Build history of the part. All positions in model axes, mm. Face numbers are marked on the shaded views. A direction names the side the tool comes from. Round coordinates to 2 decimals unless told otherwise and drop trailing zeros. Write each loop counter-clockwise with the first axis right and the second up, starting at its lowest first coordinate (ties: lowest second). Pieces come first, ordered by that corner, then holes.
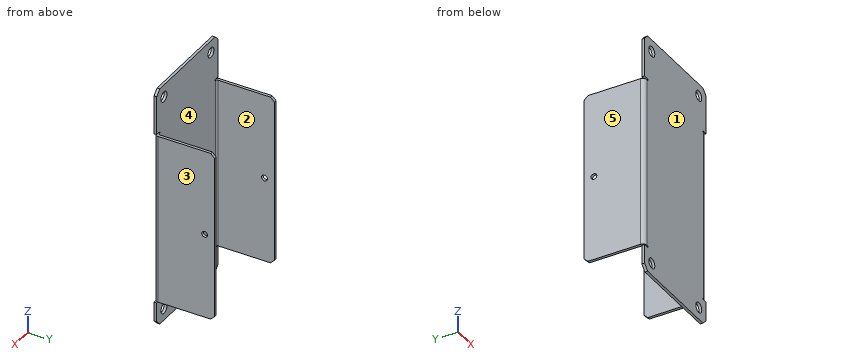
from build123d import *

# Parameters (mm, degrees)
SKETCH1_W                       = 53.65
SKETCH1_H                       = 124.45
SKETCH1_R                       = 2.61
BASE_FLANGE1_DEPTH              = 1.4
CHAMFER1_SIZE                   = 2.7
EDGE_FLANGE2_STRIP_W            = 7.0732
EDGE_FLANGE2_STRIP_H            = 1.4
EDGE_FLANGE2_STRIP_CUT_DEPTH    = 87.7
EDGE_FLANGE2_RELIEF_W           = 7.7732
EDGE_FLANGE2_RELIEF_H           = 0.7
EDGE_FLANGE2_RELIEF_CUT_DEPTH   = 1.4
EDGE_FLANGE2_STRIP_2_W          = 7.0732
EDGE_FLANGE2_STRIP_2_H          = 1.4
EDGE_FLANGE2_STRIP_CUT_2_DEPTH  = 87.7
EDGE_FLANGE2_RELIEF_2_W         = 7.7732
EDGE_FLANGE2_RELIEF_2_H         = 0.7
EDGE_FLANGE2_RELIEF_CUT_2_DEPTH = 1.4
EDGE_FLANGE2_DEPTH              = 87.7
EDGE_FLANGE2_BEND_DEPTH         = 87.7
CHAMFER2_SIZE                   = 2
SKETCH18_R                      = 1.5
CUT_EXTRUDE1_DEPTH              = 88.329451647


# Sheet-metal steps are written as plain solids
with BuildPart() as part:
    # Sketch1 → Base-Flange1 (new body)
    with BuildSketch(Plane(origin=(0, 0, 0), x_dir=(1, 0, 0), z_dir=(0, 1, 0))):
        Rectangle(SKETCH1_W, SKETCH1_H)
        with Locations(Location((-20.5, 56, 0), (0, 0, 270))):
            Circle(SKETCH1_R, mode=Mode.SUBTRACT)
        with Locations(Location((20.5, 56, 0), (0, 0, 270))):
            Circle(SKETCH1_R, mode=Mode.SUBTRACT)
        with Locations(Location((20.5, -56, 0), (0, 0, 270))):
            Circle(SKETCH1_R, mode=Mode.SUBTRACT)
        with Locations(Location((-20.5, -56, 0), (0, 0, 270))):
            Circle(SKETCH1_R, mode=Mode.SUBTRACT)
    extrude(amount=-BASE_FLANGE1_DEPTH)

    # Chamfer1
    chamfer1_edges = [part.edges().sort_by_distance(p)[0] for p in [
        (26.825, -0.7, 62.225),
        (-26.825, -0.7, 62.225),
        (-26.825, -0.7, -62.225),
        (26.825, -0.7, -62.225),
    ]]
    chamfer(chamfer1_edges, length=CHAMFER1_SIZE)

    # Edge-Flange2 strip (across the edge) → Edge-Flange2 strip cut (cut)
    with BuildSketch(Plane(origin=(26.825, 0, 38.825), x_dir=(-1, 0, 0), z_dir=(0, 0, -1))):
        with Locations((-1.4, -0.7)):
            Rectangle(EDGE_FLANGE2_STRIP_W, EDGE_FLANGE2_STRIP_H)
    extrude(amount=EDGE_FLANGE2_STRIP_CUT_DEPTH, mode=Mode.SUBTRACT)

    # Edge-Flange2 relief (on the sheet) → Edge-Flange2 relief cut (cut)
    with BuildSketch(Plane(origin=(24.6884, 0, 38.825), x_dir=(-1, 0, 0), z_dir=(0, 1, 0))):
        with Locations((-3.1866, 0.35)):
            Rectangle(EDGE_FLANGE2_RELIEF_W, EDGE_FLANGE2_RELIEF_H)
        with Locations((-3.1866, -88.05)):
            Rectangle(EDGE_FLANGE2_RELIEF_W, EDGE_FLANGE2_RELIEF_H)
    extrude(amount=-EDGE_FLANGE2_RELIEF_CUT_DEPTH, mode=Mode.SUBTRACT)

    # Edge-Flange2 strip 2 (across the edge) → Edge-Flange2 strip cut 2 (cut)
    with BuildSketch(Plane(origin=(-26.825, 0, -48.875), x_dir=(1, 0, 0), z_dir=(0, 0, 1))):
        with Locations((-1.4, -0.7)):
            Rectangle(EDGE_FLANGE2_STRIP_2_W, EDGE_FLANGE2_STRIP_2_H)
    extrude(amount=EDGE_FLANGE2_STRIP_CUT_2_DEPTH, mode=Mode.SUBTRACT)

    # Edge-Flange2 relief 2 (on the sheet) → Edge-Flange2 relief cut 2 (cut)
    with BuildSketch(Plane(origin=(-24.6884, 0, -48.875), x_dir=(1, 0, 0), z_dir=(0, 1, 0))):
        with Locations((-3.1866, 0.35)):
            Rectangle(EDGE_FLANGE2_RELIEF_2_W, EDGE_FLANGE2_RELIEF_2_H)
        with Locations((-3.1866, -88.05)):
            Rectangle(EDGE_FLANGE2_RELIEF_2_W, EDGE_FLANGE2_RELIEF_2_H)
    extrude(amount=-EDGE_FLANGE2_RELIEF_CUT_2_DEPTH, mode=Mode.SUBTRACT)

    # Edge-Flange2 section (across the edge) → Edge-Flange2 (add)
    with BuildSketch(Plane(origin=(26.825, 0, 38.825), x_dir=(-1, 0, 0), z_dir=(0, 0, -1))):
        with BuildLine():
            Line((0, 0.7366), (0, 29.6))
            Line((0, 29.6), (1.4, 29.6))
            Line((1.4, 29.6), (1.4, 0.7366))
            ThreePointArc((1.4, 0.7366), (1.615745145, 0.215745145), (2.1366, 0))
            Line((2.1366, 0), (2.1366, -1.4))
            ThreePointArc((2.1366, -1.4), (0.625795651, -0.774204349), (0, 0.7366))
        make_face()
    extrude(amount=EDGE_FLANGE2_DEPTH)

    # Edge-Flange2 section 2 (across the edge) → Edge-Flange2 bend (add)
    with BuildSketch(Plane(origin=(-26.825, 0, -48.875), x_dir=(1, 0, 0), z_dir=(0, 0, 1))):
        with BuildLine():
            Line((0, 0.7366), (0, 29.6))
            Line((0, 29.6), (1.4, 29.6))
            Line((1.4, 29.6), (1.4, 0.7366))
            ThreePointArc((1.4, 0.7366), (1.615745145, 0.215745145), (2.1366, 0))
            Line((2.1366, 0), (2.1366, -1.4))
            ThreePointArc((2.1366, -1.4), (0.625795651, -0.774204349), (0, 0.7366))
        make_face()
    extrude(amount=EDGE_FLANGE2_BEND_DEPTH)

    # Chamfer2
    chamfer2_edges = [part.edges().sort_by_distance(p)[0] for p in [
        (26.125, 29.6, 38.825),
        (26.125, 29.6, -48.875),
        (-26.125, 29.6, -48.875),
        (-26.125, 29.6, 38.825),
    ]]
    chamfer(chamfer2_edges, length=CHAMFER2_SIZE)

    # Sketch18 → Cut-Extrude1 (cut, through all)
    with BuildSketch(Plane(origin=(26.825, 0, 0), x_dir=(0, 0, -1), z_dir=(1, 0, 0))):
        with Locations(Location((5.025, 24.54, 0), (0, 0, 90))):
            Circle(SKETCH18_R)
    extrude(amount=-CUT_EXTRUDE1_DEPTH, mode=Mode.SUBTRACT)


solid = part.part
1) Slice it at D-D (y = 24.54). Write the cut outline in (x, z) (3 decimals).
Results:
outline: (-26.825, -48.875) - (-25.425, -48.875) - (-25.425, -6.525) - (-26.825, -6.525) - close; (-26.825, -3.525) - (-25.425, -3.525) - (-25.425, 38.825) - (-26.825, 38.825) - close; (25.425, -48.875) - (26.825, -48.875) - (26.825, -6.525) - (25.425, -6.525) - close; (25.425, -3.525) - (26.825, -3.525) - (26.825, 38.825) - (25.425, 38.825) - close
2) Slice it at B-B (z = -56). Write the cut outline in (x, y) (3 decimals), plus the area to 3 significant figures.
Results:
outline: (-26.825, -1.4) - (-23.11, -1.4) - (-23.11, 0) - (-26.825, 0) - close; (-17.89, -1.4) - (17.89, -1.4) - (17.89, 0) - (-17.89, 0) - close; (23.11, -1.4) - (26.825, -1.4) - (26.825, 0) - (23.11, 0) - close
area: 60.5 mm2
3) Slice it at C-C (y = 14.5). Write the cut outline in (x, z) (3 decimals), plus the area to 3 significant figures.
Results:
outline: (-26.825, -48.875) - (-25.425, -48.875) - (-25.425, 38.825) - (-26.825, 38.825) - close; (25.425, -48.875) - (26.825, -48.875) - (26.825, 38.825) - (25.425, 38.825) - close
area: 246 mm2
4) Wall check: L1, parallel to X at y = -1, z = -56 (3 decimals); L2, parallel to X at y = 27.5, z = -22 (3 decimals); L3, parallel to Y at x = 2, z = -38. Give the ranges that are in metal, low to high.
Results:
L1: x = -26.825 to -23.11, -17.89 to 17.89, 23.11 to 26.825
L2: x = -26.825 to -25.425, 25.425 to 26.825
L3: y = -1.4 to 0
5) Which spindle directions (+Z, -Z, +X, -X, +Y, -Y) get a long thin tool onto all of the face, cutting with end or side? Do the marked faces 1 and 2. Say none if no direction does.
Results:
face 1: +Z, -Z, +X, -X, -Y
face 2: +Z, -Z, +Y
6) Mould opens along X. For the marked faces 3, 4 and 5 say: released by +X, released by -X, zero draft, split by the parting line, or undercut.
Results:
face 3: released by +X
face 4: undercut
face 5: released by -X
7) Pin check, flat tips, straight feed: pin 1 Ø0.7 at (x, y) = (25.5, -0.5) entering from -Z; pin 2 Ø0.7 at (x, y) = (25.5, -0.5) entering from +Z; pin 3 Ø0.9 at (x, y) = (25.5, 9) entering from -Z (3 decimals). Stop position of each tip, or through.
Results:
pin 1: stops at z = -61.2
pin 2: stops at z = 61.2
pin 3: stops at z = -48.875
8) Slice it at A-A (x = -20.5). Write the cut outline in (y, z) (3 decimals).
Results:
outline: (-1.4, -62.225) - (0, -62.225) - (0, -58.61) - (-1.4, -58.61) - close; (-1.4, -53.39) - (0, -53.39) - (0, 53.39) - (-1.4, 53.39) - close; (-1.4, 58.61) - (0, 58.61) - (0, 62.225) - (-1.4, 62.225) - close
